Study the drawing (mm; zero at the part's minimum x, y, z) and answer. Round coordinates to 2 decimals unless told otherwise and drop trailing zeros. Order: outer loops, then holes, each group sorted by start corner. A loop starts at its lowest first (then second) coordinate and runs counter-clockwise, first axis right, second up. Notation, with made-up numbers: M -37,-8.75 L -30,-8.75 A29 ccw -30,11.25 Z; hole C -8,14.5 d3. An arc over 180 degrees is marked long. Put each result on its own line as item: value. Start each with the question number.
1. Consider line 1 (X direction, y = 1.45, z = 36); line 2 (X direction, y = 1.8, z = 13.5); line 3 (Z direction, x = 5.5, y = 2). Determine where each line is inside the solid, lowest interval first.
2. The part is cut by section C-C (y = 1.65). Give the vertices of the cut face in (x, z).
3. Each of these flat-tipped pins is pushed along its axis until it touches: pin 1 Ø2 at (x, z) = (10, 22) entering from +Y; pin 2 Ø1.5 at (x, y) = (6, 2.5) entering from +Z. Where does it stop, or does it pass through?
4. The part is cut by section D-D (x = 6). Give the vertices of the cut face in (y, z), then the cut area to 3 significant figures.
5. The part is cut by section B-B (z = 13.5). Give the vertices of the cut face in (x, y), then the cut area to 3 significant figures.
6. The part is cut by section A-A (x = 10). Give the vertices of the cut face in (y, z), then the cut area to 3 significant figures.
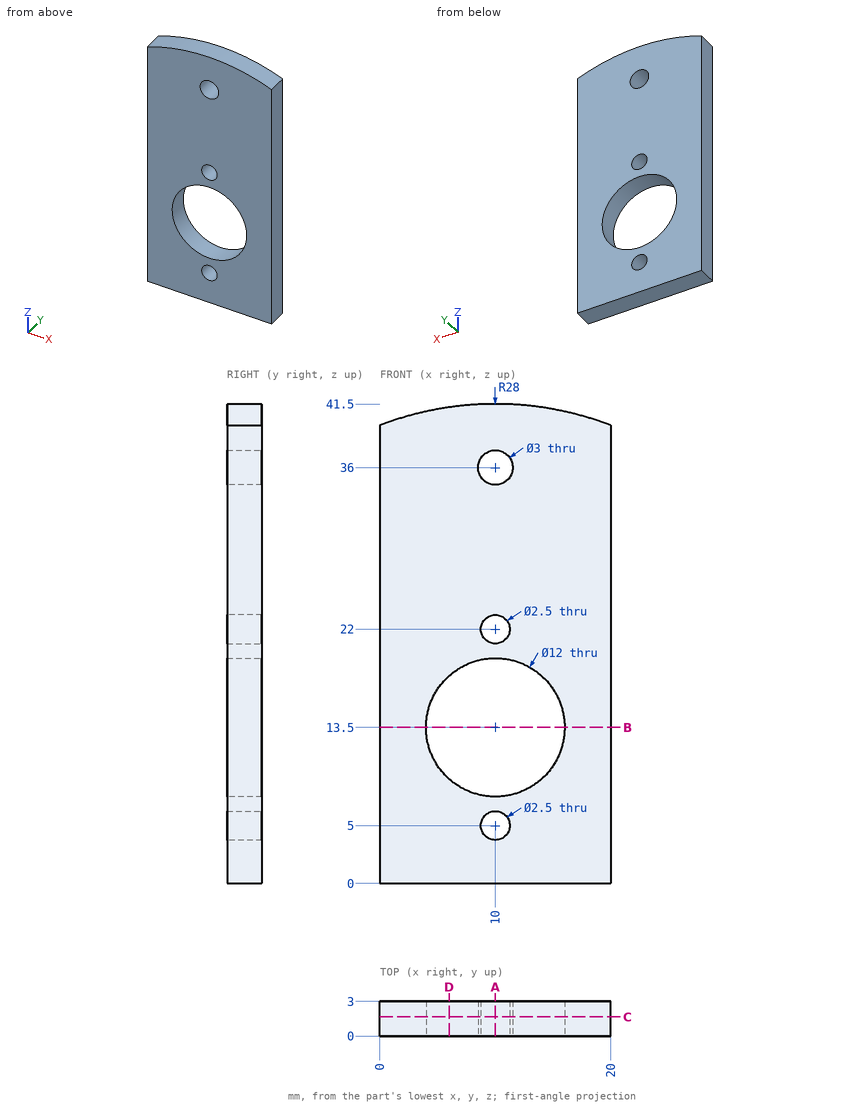
Resolved:
1. line 1: 0 to 8.5, 11.5 to 20
1. line 2: 0 to 4, 16 to 20
1. line 3: 0 to 9.53, 17.47 to 41.14
2. outline: M 0,0 L 20,0 L 20,39.65 A28 ccw 0,39.65 Z; hole C 10,13.5 d12; hole C 10,36 d3; hole C 10,5 d2.5; hole C 10,22 d2.5
3. pin 1: through
3. pin 2: z = 41.31
4. outline: M 0,0 L 3,0 L 3,9.03 L 0,9.03 Z; M 0,17.97 L 3,17.97 L 3,41.21 L 0,41.21 Z
4. area: 96.8 mm2
5. outline: M 0,0 L 4,0 L 4,3 L 0,3 Z; M 16,0 L 20,0 L 20,3 L 16,3 Z
5. area: 24.0 mm2
6. outline: M 0,0 L 3,0 L 3,3.75 L 0,3.75 Z; M 0,6.25 L 3,6.25 L 3,7.5 L 0,7.5 Z; M 0,19.5 L 3,19.5 L 3,20.75 L 0,20.75 Z; M 0,23.25 L 3,23.25 L 3,34.5 L 0,34.5 Z; M 0,37.5 L 3,37.5 L 3,41.5 L 0,41.5 Z
6. area: 64.5 mm2
